Can you work these out from the model? Positions are in its coordinate system, mm. A direction names the side the tool comes from. Give positions to 0.01 mm unless a question says otherwise; leave off trailing zeros. Order: outer loops, then holes, each group sorted by start corner. A loop starts at its lowest first (then second) coordinate and runs counter-clockwise, first axis right, second up. Notation, with made-up numbers: (17, 55) - (42, 55) arc R10 cw to (42, 66) - close; hole circle Ø5 at (22.5, 24). An arc over 180 degrees is marked (long way). One line per question, with ' | ' between items.
```python
from build123d import *

# Parameters (mm, degrees)
F0_R     = 6.75
F1_DEPTH = 2
F2_R     = 4
F3_DEPTH = 62
F4_R     = 0.25
F5_DEPTH = 29
F6_SIZE  = 0.25


with BuildPart() as f1:
    # F0 (on Top) → F1 (new body)
    with BuildSketch(Plane.XY):
        Circle(F0_R)
    extrude(amount=F1_DEPTH)

    # F2 (on face) → F3 (join)
    with BuildSketch(Plane(origin=(0, 0, 0), x_dir=(1, 0, 0), z_dir=(0, 0, -1))):
        Circle(F2_R)
    extrude(amount=F3_DEPTH)

    # F4 (on face) → F5 (join)
    with BuildSketch(Plane(origin=(0, 0, -62), x_dir=(1, 0, 0), z_dir=(0, 0, -1))):
        Circle(F4_R)
    extrude(amount=F5_DEPTH)

    # F6
    f6_edges = [f1.edges().sort_by_distance(p)[0] for p in [
        (-0.25, 0, -91),
    ]]
    chamfer(f6_edges, length=F6_SIZE)


solid = f1.part
```
(1) Imagine slicing it at C-C (y = -1.75). List the corners of the cut face in (x, z) for me.
Answer below:
outline: (-6.52, 0) - (-3.6, 0) - (-3.6, -62) - (3.6, -62) - (3.6, 0) - (6.52, 0) - (6.52, 2) - (-6.52, 2) - close
(2) Imagine slicing it at B-B (x = -2). List the corners of the cut face in (y, z) for me.
Answer below:
outline: (-6.45, 0) - (-3.46, 0) - (-3.46, -62) - (3.46, -62) - (3.46, 0) - (6.45, 0) - (6.45, 2) - (-6.45, 2) - close
(3) On a 3-axis mill with a long thin cutter (end or side, diameter ignored), from which of +Z, -Z, +X, -X, +Y, -Y can I reach the whole of each face in a straight line? I mean faces 1 (the face through (0, 0, 2)), 2 (the face through (3, -3, 0)). Say none if no direction works.
Answer below:
face 1: +Z, +X, -X, +Y, -Y | face 2: -Z
(4) Imagine slicing it at D-D (z = -80). List the corners of the cut face in (x, y) for me.
Answer below:
outline: circle Ø0.5 at (0, 0)
(5) Will these pins go through, and if not, where does the flat tip stop? pin 1 (2 mm diameter, centred on x = 4, z = -29.5, fed in from -Y); pin 2 (2.5 mm diameter, centred on x = 0, y = -0.5, fed in from -Z); pin 3 (8 mm diameter, centred on y = 1.5, z = -15, fed in from +X); pin 4 (5 mm diameter, centred on x = 5, y = -3, fed in from -Z).
Answer below:
pin 1: y = -2.65 | pin 2: z = -91 | pin 3: x = 4 | pin 4: z = -62
(6) If I drill on line 1 (Z direction, x = 5.25, y = -4); line 2 (Z direction, x = 1.25, y = 2); line 3 (Y direction, x = 2.5, z = -19.5), over which ranges is the centre line in solid material (lowest first)?
Answer below:
line 1: 0 to 2 | line 2: -62 to 2 | line 3: -3.12 to 3.12
(7) Imagine slicing it at A-A (z = -54). List the corners of the cut face in (x, y) for me.
Answer below:
outline: circle Ø8 at (0, 0)
